Job drawing, mm, ordinate dimensions from the low corner. One solid piece. A direction names the side the tool comes from. Give positions to 0.01 mm unless a question says otherwise; leave off trailing zeros. Order: outer loops, then holes, each group sorted by start corner. A loop starts at its lowest first (then second) coordinate and runs counter-clockwise, first axis right, second up.
Item 1: Band-saw the part on B-B on y = 73. Give the cut face in (x, z).
Item 2: Which spindle directions (+Z, -Z, +X, -X, +Y, -Y) get a long thin tool onto all of the face, cutting with end or side? Do the marked faces 1 and 2. Say none if no direction does.
Item 3: Wall check: L1, parallel to X at y = 20, z = 4.55; L2, parallel to Z at x = 21.25, y = 63; L3, parallel to X at y = 25.5, z = 2.4. Give the ranges that are in metal, low to high.
Item 4: Flat gauge pin, fed straight in: P1, Ø4, axis at x = 14.5, y = 27, coming from the +Z side. Where does the tip first touch, or does it go through?
Item 5: Band-saw the part on C-C on x = 13.5. Give the cut face in (y, z), plus the area to 3 significant figures.
Item 6: Band-saw the part on A-A on z = 3.7. Give the cut face in (x, y).
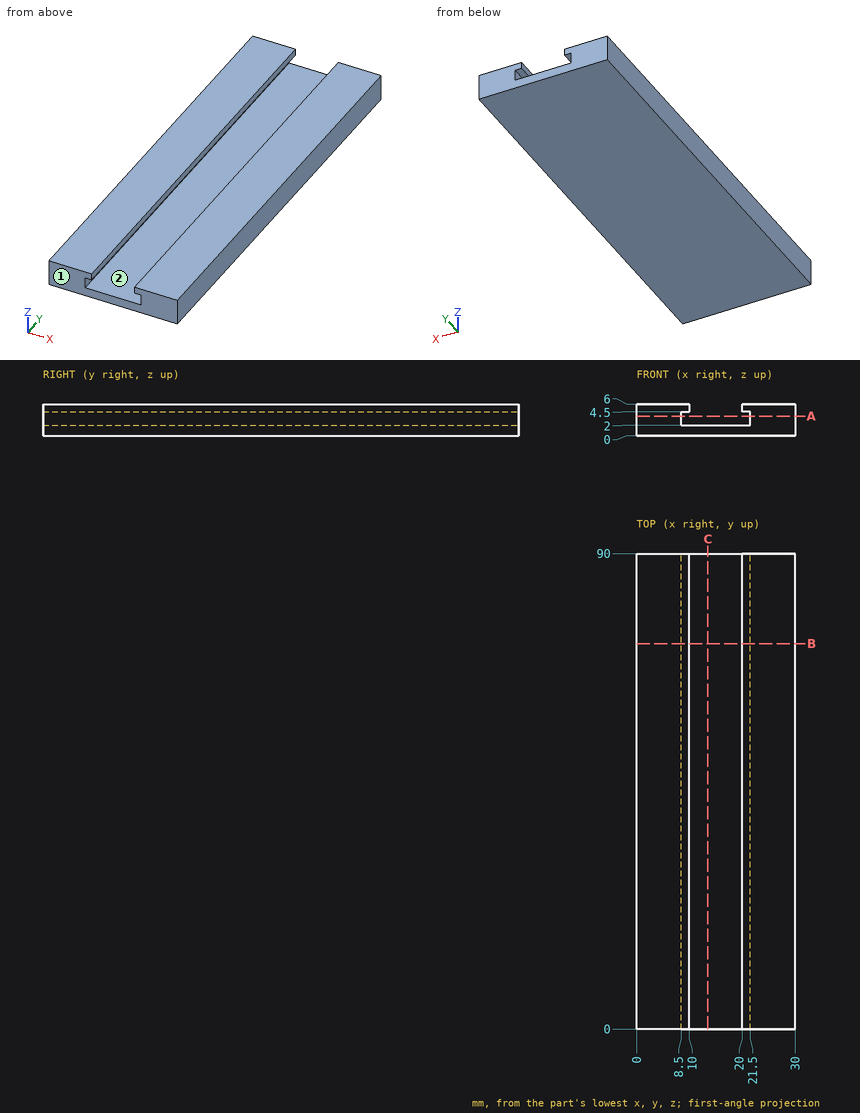
The answers:
1. outline: (0, 0) - (30, 0) - (30, 6) - (20, 6) - (20, 4.5) - (21.5, 4.5) - (21.5, 2) - (8.5, 2) - (8.5, 4.5) - (10, 4.5) - (10, 6) - (0, 6) - close
2. face 1: +Z, -Z, +X, -X, -Y
2. face 2: +Y, -Y
3. L1: x = 0 to 10, 20 to 30
3. L2: z = 0 to 2, 4.5 to 6
3. L3: x = 0 to 8.5, 21.5 to 30
4. P1: stops at z = 2
5. outline: (0, 0) - (90, 0) - (90, 2) - (0, 2) - close
5. area: 180 mm2
6. outline: (0, 0) - (8.5, 0) - (8.5, 90) - (0, 90) - close; (21.5, 0) - (30, 0) - (30, 90) - (21.5, 90) - close
